Geometry: final body of the model. Coordinates: model frame, mm. Face numbers are marked on the shaded views. Give positions to 0.01 mm unless a question says otherwise; leave off trailing zeros. Order: outer loops, then holes, each group sorted by start corner. A loop starts at its lowest first (then second) coordinate and runs counter-clockwise, first axis right, second up. Notation, with made-up numbers: (-13.5, 41) -> (2.5, 41) arc R9 cw to (2.5, 46) -> close; hole circle Ø5 at (-26.5, -33). An arc over 180 degrees is marked (long way). One line per item, written item: value. Start each with the question number.
```python
from build123d import *

# Parameters (mm, degrees)
F1_W      = 59.69
F1_H      = 28.575
F1_R      = 1.5748
F1_R_2    = 0.79375
F2_DEPTH  = 2.54
F3_W      = 5.600192
F3_H      = 7.500214
F4_DEPTH  = 2.54
F5_W      = 16.800018
F5_H      = 3.139999
F6_DEPTH  = 2.921
F7_W      = 4.826
F7_H      = 2.4892
F7_W_2    = 4.2418
F7_H_2    = 3.2512
F8_DEPTH  = 2.286
F9_R      = 0.4445
F10_DEPTH = 6.096
F11_W     = 35.306
F11_H     = 10.16
F12_DEPTH = 2.286
F13_R     = 0.4445
F14_DEPTH = 5.969


with BuildPart() as f2:
    # F1 (on Top) → F2 (new body)
    with BuildSketch(Plane.XY):
        with Locations((-0.701548, 0)):
            Rectangle(F1_W, F1_H)
        with Locations((-27.371548, -11.2395)):
            Circle(F1_R, mode=Mode.SUBTRACT)
        with Locations((9.331452, -9.4615)):
            Circle(F1_R_2, mode=Mode.SUBTRACT)
        with Locations((14.538452, -11.2395)):
            Circle(F1_R, mode=Mode.SUBTRACT)
        with Locations((-27.371548, 11.1125)):
            Circle(F1_R, mode=Mode.SUBTRACT)
        with Locations((-19.370548, 11.1125)):
            Circle(F1_R_2, mode=Mode.SUBTRACT)
        with Locations((14.538452, 11.1125)):
            Circle(F1_R, mode=Mode.SUBTRACT)
    extrude(amount=F2_DEPTH)

    # F3 (on face) → F4 (join)
    with BuildSketch(Plane.XY.offset(2.54)):
        with Locations((27.619452, 8.8265)):
            Rectangle(F3_W, F3_H)
        with Locations((27.746452, -3.6195)):
            Rectangle(F3_W, F3_H)
    extrude(amount=F4_DEPTH)

    # F5 (on face) → F6 (join)
    with BuildSketch(Plane.XY.offset(2.54)):
        with Locations((-1.058545, -8.963304)):
            Rectangle(F5_W, F5_H)
    extrude(amount=F6_DEPTH)

    # F7 (on face) → F8 (join)
    with BuildSketch(Plane.XY.offset(2.54)):
        with Locations((26.349452, -11.4935)):
            Rectangle(F7_W, F7_H)
        with Locations((-27.244548, 6.2865)):
            Rectangle(F7_W, F7_H)
        with Locations((-27.117548, 2.4765)):
            Rectangle(F7_W, F7_H)
        with Locations((-27.117548, -5.9055)):
            Rectangle(F7_W_2, F7_H_2)
    extrude(amount=F8_DEPTH)

    # F9 (on face) → F10 (join)
    with BuildSketch(Plane.XY.offset(4.826)):
        with Locations((-28.514548, 6.2865)):
            Circle(F9_R)
        with Locations((-25.974548, 6.2865)):
            Circle(F9_R)
        with Locations((-28.387548, 2.4765)):
            Circle(F9_R)
        with Locations((-25.974548, 2.4765)):
            Circle(F9_R)
        with Locations((27.619452, -11.4935)):
            Circle(F9_R)
        with Locations((25.079452, -11.4935)):
            Circle(F9_R)
    extrude(amount=F10_DEPTH)

    # F11 (on face) → F12 (join)
    with BuildSketch(Plane.XY):
        with Locations((-5.400548, 2.4765)):
            Rectangle(F11_W, F11_H)
    extrude(amount=-F12_DEPTH)

    # F13 (on face) → F14 (join)
    with BuildSketch(Plane(origin=(0, 0, -2.286), x_dir=(1, 0, 0), z_dir=(0, 0, -1))):
        with Locations((-21.783548, 1.3335)):
            Circle(F13_R)
        with Locations((-19.243548, 1.3335)):
            Circle(F13_R)
        with Locations((-16.703548, 1.3335)):
            Circle(F13_R)
        with Locations((-14.163548, 1.3335)):
            Circle(F13_R)
        with Locations((-11.623548, 1.3335)):
            Circle(F13_R)
        with Locations((-9.083548, 1.3335)):
            Circle(F13_R)
        with Locations((-6.543548, 1.3335)):
            Circle(F13_R)
        with Locations((-4.003548, 1.3335)):
            Circle(F13_R)
        with Locations((-1.463548, 1.3335)):
            Circle(F13_R)
        with Locations((1.076452, 1.3335)):
            Circle(F13_R)
        with Locations((3.616452, 1.3335)):
            Circle(F13_R)
        with Locations((6.156452, 1.3335)):
            Circle(F13_R)
        with Locations((8.696452, 1.3335)):
            Circle(F13_R)
        with Locations((11.236452, 1.3335)):
            Circle(F13_R)
        with Locations((-21.783548, -1.219218)):
            Circle(F13_R)
        with Locations((-19.243548, -1.219218)):
            Circle(F13_R)
        with Locations((-16.703548, -1.219218)):
            Circle(F13_R)
        with Locations((-14.163548, -1.219218)):
            Circle(F13_R)
        with Locations((-11.623548, -1.219218)):
            Circle(F13_R)
        with Locations((-9.083548, -1.219218)):
            Circle(F13_R)
        with Locations((-6.543548, -1.219218)):
            Circle(F13_R)
        with Locations((-4.003548, -1.219218)):
            Circle(F13_R)
        with Locations((-1.463548, -1.219218)):
            Circle(F13_R)
        with Locations((1.076452, -1.219218)):
            Circle(F13_R)
        with Locations((3.616452, -1.219218)):
            Circle(F13_R)
        with Locations((6.156452, -1.219218)):
            Circle(F13_R)
        with Locations((8.696452, -1.219218)):
            Circle(F13_R)
        with Locations((11.236452, -1.219218)):
            Circle(F13_R)
        with Locations((-21.783548, -3.771936)):
            Circle(F13_R)
        with Locations((-19.243548, -3.771936)):
            Circle(F13_R)
        with Locations((-16.703548, -3.771936)):
            Circle(F13_R)
        with Locations((-14.163548, -3.771936)):
            Circle(F13_R)
        with Locations((-11.623548, -3.771936)):
            Circle(F13_R)
        with Locations((-9.083548, -3.771936)):
            Circle(F13_R)
        with Locations((-6.543548, -3.771936)):
            Circle(F13_R)
        with Locations((-4.003548, -3.771936)):
            Circle(F13_R)
        with Locations((-1.463548, -3.771936)):
            Circle(F13_R)
        with Locations((1.076452, -3.771936)):
            Circle(F13_R)
        with Locations((3.616452, -3.771936)):
            Circle(F13_R)
        with Locations((6.156452, -3.771936)):
            Circle(F13_R)
        with Locations((8.696452, -3.771936)):
            Circle(F13_R)
        with Locations((11.236452, -3.771936)):
            Circle(F13_R)
        with Locations((-21.783548, -6.324655)):
            Circle(F13_R)
        with Locations((-19.243548, -6.324655)):
            Circle(F13_R)
        with Locations((-16.703548, -6.324655)):
            Circle(F13_R)
        with Locations((-14.163548, -6.324655)):
            Circle(F13_R)
        with Locations((-11.623548, -6.324655)):
            Circle(F13_R)
        with Locations((-9.083548, -6.324655)):
            Circle(F13_R)
        with Locations((-6.543548, -6.324655)):
            Circle(F13_R)
        with Locations((-4.003548, -6.324655)):
            Circle(F13_R)
        with Locations((-1.463548, -6.324655)):
            Circle(F13_R)
        with Locations((1.076452, -6.324655)):
            Circle(F13_R)
        with Locations((3.616452, -6.324655)):
            Circle(F13_R)
        with Locations((6.156452, -6.324655)):
            Circle(F13_R)
        with Locations((8.696452, -6.324655)):
            Circle(F13_R)
        with Locations((11.236452, -6.324655)):
            Circle(F13_R)
    extrude(amount=F14_DEPTH)


solid = f2.part
```
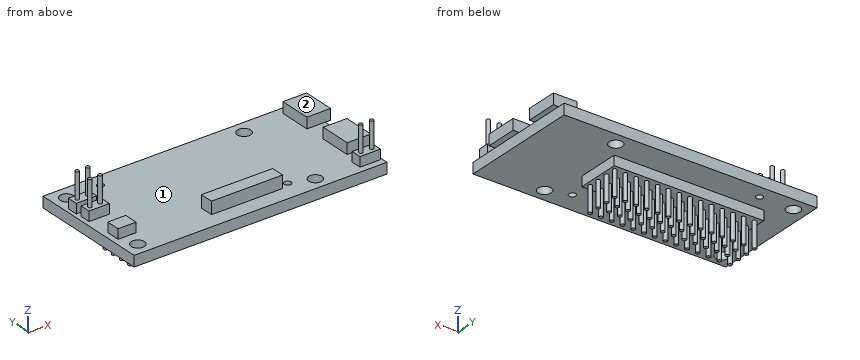
1. Cut plane B-B, the plane y = 8.75. Return loops of the section in (x, z), then the cut area to 3 significant figures.
2. Cut plane C-C, the plane x = -13. Return loops of the section in (y, z).
3. Cut plane D-D, the plane z = 8. Return loops of the section in (x, y).
4. Draft query along X for the marked faces 1 and 2. Return one class per face: pulls with the +X half, pulls with the -X half, needs draft (parallel to the pull), parting line crosses it, or undercut.
5. Material intervals for L1, parallel to Y at x = 11.5, z = -4.25; L2, parallel to Z at x = -8.5, y = 0; L3, parallel to X at y = 3, z = 2.25, sorted ascending. Write a range as [from, to].
6. Cut plane A-A, the plane z = 3.5. Return loops of the section in (x, y), then the cut area to 3 significant figures.
7. Pin query (flat end, axial travel): P1, Ø4, axis at x = -3.5, y = -10, coming from the +Z side; P2, Ø2, axis at y = 8.5, z = 4, coming from the +X side; P3, Ø1.3, axis at x = 26.5, z = 3.5, coming from the -Y side. Return the tip coordinate at first contact, or that it passes through.
Answers follow:
1. outline: (-30.55, 0) -> (29.14, 0) -> (29.14, 2.54) -> (30.42, 2.54) -> (30.42, 5.08) -> (24.82, 5.08) -> (24.82, 2.54) -> (-30.55, 2.54) -> close
1. area: 166 mm²
2. outline: (-14.29, 0) -> (-2.6, 0) -> (-2.6, -2.29) -> (7.56, -2.29) -> (7.56, 0) -> (14.29, 0) -> (14.29, 2.54) -> (-14.29, 2.54) -> close
3. outline: circle Ø0.89 at (-28.51, 6.29); circle Ø0.89 at (-28.39, 2.48); circle Ø0.89 at (-25.97, 2.48); circle Ø0.89 at (-25.97, 6.29); circle Ø0.89 at (25.08, -11.49); circle Ø0.89 at (27.62, -11.49)
4. face 1: undercut
4. face 2: needs draft
5. L1: y = [-1.69, -0.98], [0.86, 1.58], [3.41, 4.13], [5.97, 6.68]
5. L2: z = [-2.29, 2.54]
5. L3: x = [-30.55, 29.14]
6. outline: (-29.66, 5.04) -> (-24.83, 5.04) -> (-24.83, 7.53) -> (-29.66, 7.53) -> close; (-29.53, 1.23) -> (-24.7, 1.23) -> (-24.7, 3.72) -> (-29.53, 3.72) -> close; (-29.24, -7.53) -> (-25, -7.53) -> (-25, -4.28) -> (-29.24, -4.28) -> close; (-9.46, -10.53) -> (7.34, -10.53) -> (7.34, -7.39) -> (-9.46, -7.39) -> close; (23.94, -12.74) -> (28.76, -12.74) -> (28.76, -10.25) -> (23.94, -10.25) -> close; (24.82, 5.08) -> (30.42, 5.08) -> (30.42, 12.58) -> (24.82, 12.58) -> close; (24.95, -7.37) -> (30.55, -7.37) -> (30.55, 0.13) -> (24.95, 0.13) -> close
6. area: 187 mm²
7. P1: stops at z = 5.46
7. P2: stops at x = 30.42
7. P3: stops at y = -12.74
